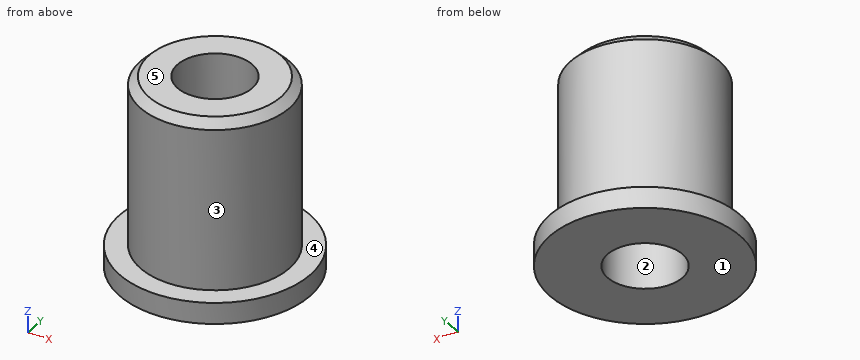
from build123d import *

# Parameters (mm, degrees)
F0_R     = 28.575
F1_DEPTH = 6.35
F2_R     = 22.352
F3_DEPTH = 50.8
F4_R     = 11.2395
F5_DEPTH = 57.151
F6_SIZE  = 2.54


with BuildPart() as f1:
    # F0 (on Top) → F1 (new body)
    with BuildSketch(Plane.XY):
        Circle(F0_R)
    extrude(amount=F1_DEPTH)

    # F2 (on face) → F3 (join)
    with BuildSketch(Plane.XY.offset(6.35)):
        Circle(F2_R)
    extrude(amount=F3_DEPTH)

    # F4 (on face) → F5 (cut, through all)
    with BuildSketch(Plane.XY.offset(57.15)):
        Circle(F4_R)
    extrude(amount=-F5_DEPTH, mode=Mode.SUBTRACT)

    # F6
    f6_edges = [f1.edges().sort_by_distance(p)[0] for p in [
        (-22.352, 0, 57.15),
    ]]
    chamfer(f6_edges, length=F6_SIZE)


solid = f1.part
The model under review builds one solid part; all positions refer to its coordinate system, in mm. Face numbers are marked on the shaded views. A direction names the side the tool comes from. Give positions to 0.01 mm unless a question says otherwise; leave off trailing zeros. Order: outer loops, then holes, each group sorted by start corner. A loop starts at its lowest first (then second) coordinate and runs counter-clockwise, first axis right, second up. Notation, with made-up numbers: M 4.25,78 L 48.25,78 A24 cw 48.25,116 Z; hole C 24,68.5 d11. An arc over 180 degrees is marked long. Answer in a Markdown table with one row per item. Add a question column.
1. Add section D-D on y = 24. State the section outline as (x, z) points, plus the area to 3 significant figures.
2. Machinability: for the marked faces 4 and 5, which of the approach directions +Z, -Z, +X, -X, +Y, -Y give a long, thin tool a straight path to every point of the face, cutting with its end or side? Answer none if there is none.
3. Mouldability with a two-part tool opening along X and no side actions: class the marked faces 1, 2 and 3 as released by +X, released by -X, zero draft, split by the parting line, or undercut.
4. For pin 1 Ø4 at (x, z) = (14, 18.5) entering from -Y; pin 2 Ø20 at (x, y) = (0, 0) entering from -Z; pin 3 Ø10 at (x, z) = (1, 40) entering from +Y; pin 4 Ø2 at (y, z) = (9.5, 30) entering from -X, all flat-tipped, find the tip position at first contact; note any pin that passes through.
5. Add section C-C on z = 39.5. State the section outline as (x, y) points.
6. To check wall thickness, follow line 1 along Y through (x, z) = (0, 15); line 2 along Z through (x, y) = (23.5, 15); line 3 along X through (y, z) = (7, 53). State the ranges of each line that lie inside material, in increasing order.
The answers:
| question | item | result |
|---|---|---|
| 1 | outline | M -15.51,0 L 15.51,0 L 15.51,6.35 L -15.51,6.35 Z |
| 1 | area | 197 mm2 |
| 2 | face 4 | +Z |
| 2 | face 5 | +Z, +X, -X, +Y, -Y |
| 3 | face 1 | zero draft |
| 3 | face 2 | undercut |
| 3 | face 3 | split by the parting line |
| 4 | pin 1 | y = -18.86 |
| 4 | pin 2 | through |
| 4 | pin 3 | y = 22.35 |
| 4 | pin 4 | x = -20.67 |
| 5 | outline | C 0,0 d44.7; hole C 0,0 d22.48 |
| 6 | line 1 | -22.35 to -11.24, 11.24 to 22.35 |
| 6 | line 2 | 0 to 6.35 |
| 6 | line 3 | -21.23 to -8.79, 8.79 to 21.23 |
